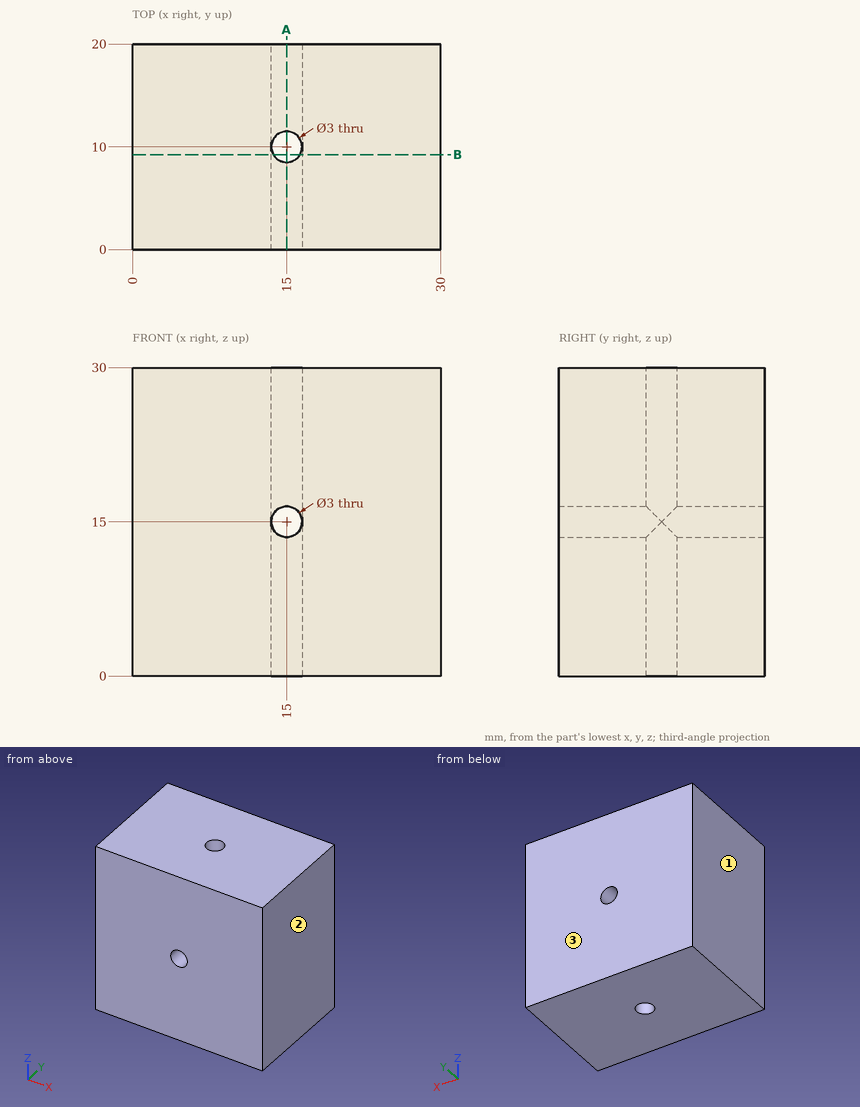
Could you check a few things on this drawing? It's one solid part, dimensions in mm from its lowest x, y, z. Give positions to 0.01 mm unless a question says otherwise; leave off trailing zeros. Write each loop counter-clockwise with the first axis right and the second up, starting at its lowest first coordinate (ties: lowest second). Pieces come first, ordered by that corner, then holes. Notation, with made-up numbers: (39, -17) -> (46, -17) arc R12 cw to (46, -5) -> close; hole circle Ø8 at (-38.5, 23.5). An arc over 180 degrees is marked (long way). Write item = value, one per line.
(1) I need wall thicknesses on probe 1 along Y at (x, z) = (15, 22.25); probe 2 along X at (y, z) = (10, 8). Which ranges of each line are inside material? Lowest first, please. Write a range as from..to.
Worked out:
probe_1 = 0..8.5, 11.5..20
probe_2 = 0..13.5, 16.5..30
(2) Suppose I cut it at B-B on y = 9.25. Write out the boundary of the cut face in (x, z), then the cut area to 3 significant figures.
Worked out:
outline = (0, 0) -> (13.7, 0) -> (13.7, 14.25) arc R1.5 cw to (13.7, 15.75) -> (13.7, 30) -> (0, 30) -> close; (16.3, 0) -> (30, 0) -> (30, 30) -> (16.3, 30) -> (16.3, 15.75) arc R1.5 cw to (16.3, 14.25) -> close
area = 822 mm^2
(3) Suppose I cut it at A-A on x = 15. Write out the boundary of the cut face in (y, z).
Worked out:
outline = (0, 0) -> (8.5, 0) -> (8.5, 13.5) -> (0, 13.5) -> close; (0, 16.5) -> (8.5, 16.5) -> (8.5, 30) -> (0, 30) -> close; (11.5, 0) -> (20, 0) -> (20, 13.5) -> (11.5, 13.5) -> close; (11.5, 16.5) -> (20, 16.5) -> (20, 30) -> (11.5, 30) -> close
(4) Thinking about a two-plate mould opening in X: for the marked faces 1, 2 and 3, which applies, released by +X, released by -X, zero draft, split by the parting line, or undercut?
Worked out:
face_1 = released by -X
face_2 = released by +X
face_3 = zero draft
